Could you check a few things on this model? Use its own coordinates, in mm. A direction names the side the tool comes from. Coordinates: 2 decimals unless noted, no trailing zeros. Loops run counter-clockwise (first coordinate to the right, second up) from the corner with the lowest first, then second, coordinate; pieces in that order, holes last.
1) Imagine slicing it at D-D on y = 33.5. Please give me the cut outline in (x, z), plus the area to 4 significant figures.
2) Imagine slicing it at C-C on z = -61. Please give me the cut outline in (x, y).
3) Imagine slicing it at A-A on x = 125.5. Please give me the cut outline in (y, z), plus the area to 3 significant figures.
4) Will these pins go through, and if not, where does the flat tip stop? P1, Ø4, axis at x = 106, z = -10, coming from the +Y side; P2, Ø2, axis at x = 74, y = 4.5, coming from the +Z side; P3, Ø5, axis at y = 26, z = -48.5, coming from the +X side; P4, Ø10, axis at x = 133, y = 25.5, coming from the -Z side.
5) Imagine slicing it at B-B on y = 23. Please give me the cut outline in (x, z), plus the area to 4 significant figures.
6) Thinking about a two-plate mould opening in X: for faces 4 (the face through (58, 5, -38)), 5 (the face through (118, 20, -41)), 6 (the face through (3, 25, -25)), 7 (the face through (60, 20, -75)), which applies, released by +X, released by -X, zero draft, split by the parting line, or undercut?
7) If I drill on line 1 along Y through (x, z) = (125.5, -1.65); line 2 along X through (y, z) = (30, -43.5); line 3 along Z through (x, y) = (79.5, 30), over which ranges is the centre line in solid material (lowest first)?
8) For faces 1 (the face through (5, 27, -50)), 2 (the face through (3, 15, -13)), 3 (the face through (128, 5, -43)), which set-ups out of +Z, -Z, +X, -X, +Y, -Y let a thin tool reach every point of the face, with its end or its side?
```python
from build123d import *

# Parameters (mm, degrees)
ESQUISSE1_W             = 138
ESQUISSE1_H             = 75
BOSS_EXTRU_1_DEPTH      = 5
ESQUISSE2_W             = 5
ESQUISSE2_H             = 75
ESQUISSE2_W_2           = 25
BOSS_EXTRU_2_DEPTH      = 30
CONG_1_R                = 13.85
ESQUISSE3_W             = 138
ESQUISSE3_H             = 35
BOSS_EXTRU_3_DEPTH      = 5
ESQUISSE4_W             = 25
ESQUISSE4_H             = 20
ENL_V_MAT_EXTRU_1_DEPTH = 6
ESQUISSE5_W             = 20
ESQUISSE5_H             = 76
ENL_V_MAT_EXTRU_2_DEPTH = 30
ESQUISSE6_R             = 6.25
ENL_V_MAT_EXTRU_3_DEPTH = 4


with BuildPart() as part:
    # Esquisse1 → Boss.-Extru.1 (new body)
    with BuildSketch(Plane(origin=(0, 0, 0), x_dir=(1, 0, 0), z_dir=(0, 1, 0))):
        with Locations((69, 37.5)):
            Rectangle(ESQUISSE1_W, ESQUISSE1_H)
    extrude(amount=BOSS_EXTRU_1_DEPTH)

    # Esquisse2 → Boss.-Extru.2 (add)
    with BuildSketch(Plane(origin=(0, 5, 0), x_dir=(1, 0, 0), z_dir=(0, 1, 0))):
        with Locations((2.5, 37.5)):
            Rectangle(ESQUISSE2_W, ESQUISSE2_H)
        with Locations((125.5, 37.5)):
            Rectangle(ESQUISSE2_W_2, ESQUISSE2_H)
    extrude(amount=BOSS_EXTRU_2_DEPTH)

    # Congé1
    cong_1_edges = [part.edges().sort_by_distance(p)[0] for p in [
        (5, 5, -37.5),
        (113, 5, -37.5),
    ]]
    fillet(cong_1_edges, radius=CONG_1_R)

    # Esquisse3 → Boss.-Extru.3 (add)
    with BuildSketch(Plane(origin=(0, 0, -75), x_dir=(-1, 0, 0), z_dir=(0, 0, -1))):
        with Locations((-69, 17.5)):
            Rectangle(ESQUISSE3_W, ESQUISSE3_H)
    extrude(amount=BOSS_EXTRU_3_DEPTH)

    # Esquisse4 → Enlèv. mat.-Extru.1 (cut)
    with BuildSketch(Plane.ZY):
        with Locations((-12.5, 25)):
            Rectangle(ESQUISSE4_W, ESQUISSE4_H)
    extrude(amount=-ENL_V_MAT_EXTRU_1_DEPTH, mode=Mode.SUBTRACT)

    # Esquisse5 → Enlèv. mat.-Extru.2 (cut)
    with BuildSketch(Plane(origin=(0, 35, 0), x_dir=(1, 0, 0), z_dir=(0, 1, 0))):
        with Locations((128, 42)):
            Rectangle(ESQUISSE5_W, ESQUISSE5_H)
    extrude(amount=-ENL_V_MAT_EXTRU_2_DEPTH, mode=Mode.SUBTRACT)

    # Esquisse6 → Enlèv. mat.-Extru.3 (cut)
    with BuildSketch(Plane.XY):
        with Locations((125.5, 23)):
            Circle(ESQUISSE6_R)
    extrude(amount=-ENL_V_MAT_EXTRU_3_DEPTH, mode=Mode.SUBTRACT)


solid = part.part
```
Filled in:
1. outline: (0, -80) - (118, -80) - (118, -4) - (138, -4) - (138, 0) - (113, 0) - (113, -75) - (5, -75) - (5, -25) - (0, -25) - close
1. area: 1,295 mm2
2. outline: (0, 0) - (138, 0) - (138, 5) - (118, 5) - (118, 35) - (113, 35) - (113, 18.85) arc R13.85 cw to (99.15, 5) - (18.85, 5) arc R13.85 cw to (5, 18.85) - (5, 35) - (0, 35) - close
3. outline: (0, -80) - (5, -80) - (5, -4) - (16.75, -4) - (16.75, 0) - (0, 0) - close; (29.25, -4) - (35, -4) - (35, 0) - (29.25, 0) - close
3. area: 470 mm2
4. P1: stops at y = 8.2
4. P2: stops at z = 0
4. P3: stops at x = 118
4. P4: stops at z = -4
5. outline: (0, -80) - (118, -80) - (118, -4) - (119.25, -4) - (119.25, 0) - (113, 0) - (113, -75) - (5, -75) - (5, -25) - (0, -25) - close; (131.75, -4) - (138, -4) - (138, 0) - (131.75, 0) - close
5. area: 1,245 mm2
6. face 4: undercut
6. face 5: released by +X
6. face 6: zero draft
6. face 7: undercut
7. line 1: y = 0 to 16.75, 29.25 to 35
7. line 2: x = 0 to 5, 113 to 118
7. line 3: z = -80 to -75
8. face 1: +Z, +Y
8. face 2: +Z, -X, +Y
8. face 3: -Z, +X, +Y
